Work out the finished part from the listing and answer in its coordinate system (mm). A direction names the side the tool comes from. Give positions to 0.01 mm unless a question says otherwise; leave off trailing zeros. Loops run counter-clockwise (first coordinate to the right, second up) from the corner with the lowest first, then second, coordinate; pieces in that order, holes last. Notation, with made-up numbers: (82, -12.5) - (112, -12.5) arc R22 cw to (112, 11.5) - close; hole circle Ø8 at (21, 26). An arc over 180 degrees is marked (long way). One line per question, with ' | ' between items. Start each with the question number.
1. For a pull along X with two mould halves and no side action, classify faces 1 (the face through (-5, -1.5, 2)), 2 (the face through (7.5, 0, 3)), 3 (the face through (0, -7.5, 3)) as released by +X, released by -X, zero draft, split by the parting line, or undercut.
2. Section B-B (z = 2.15) is taken. Determine the outline of the cut face in (x, y), plus the area to 3 significant figures.
3. Which of the six approach directions +Z, -Z, +X, -X, +Y, -Y give full straight-line access (tool end or side, diameter ignored) to faces 4 (the face through (0, 0, 6)), 5 (the face through (5.55, -3, 2))?
4. Find the intervals of material crossed by line 1 (Y direction, x = -5.5, z = 3.55); line 2 (Y direction, x = 0, z = 4.4), in increasing order.
5. Section D-D (y = 0) is taken. Determine the outline of the cut face in (x, z).
6. Section A-A (x = -5.25) is taken. Determine the outline of the cut face in (y, z).
from build123d import *

# Parameters (mm, degrees)
SKETCH1_W           = 15
SKETCH1_H           = 15
BOSS_EXTRUDE1_DEPTH = 5
SKETCH2_W           = 15
SKETCH2_H           = 15
BOSS_EXTRUDE2_DEPTH = 1


with BuildPart() as part:
    # Sketch1 → Boss-Extrude1 (new body)
    with BuildSketch(Plane.XY):
        Rectangle(SKETCH1_W, SKETCH1_H)
        Polygon((-5.55, 5.55), (-1.5, 5.55), (-1.5, 3.55), (1.5, 3.55), (1.5, 5.55), (5.55, 5.55), (5.55, 1.5), (3.55, 1.5), (3.55, -1.5), (5.55, -1.5), (5.55, -5.55), (1.5, -5.55), (1.5, -3.55), (-1.5, -3.55), (-1.5, -5.55), (-5.55, -5.55), (-5.55, -1.5), (-3.55, -1.5), (-3.55, 1.5), (-5.55, 1.5), align=None, mode=Mode.SUBTRACT)
    extrude(amount=BOSS_EXTRUDE1_DEPTH)

    # Sketch2 → Boss-Extrude2 (add)
    with BuildSketch(Plane.XY.offset(5)):
        Rectangle(SKETCH2_W, SKETCH2_H)
    extrude(amount=BOSS_EXTRUDE2_DEPTH)


solid = part.part
Conclusion:
1) face 1: undercut | face 2: released by +X | face 3: zero draft
2) outline: (-7.5, -7.5) - (7.5, -7.5) - (7.5, 7.5) - (-7.5, 7.5) - close; hole (-5.55, -5.55) - (-1.5, -5.55) - (-1.5, -3.55) - (1.5, -3.55) - (1.5, -5.55) - (5.55, -5.55) - (5.55, -1.5) - (3.55, -1.5) - (3.55, 1.5) - (5.55, 1.5) - (5.55, 5.55) - (1.5, 5.55) - (1.5, 3.55) - (-1.5, 3.55) - (-1.5, 5.55) - (-5.55, 5.55) - (-5.55, 1.5) - (-3.55, 1.5) - (-3.55, -1.5) - (-5.55, -1.5) - close | area: 126 mm²
3) face 4: +Z, +X, -X, +Y, -Y | face 5: -Z
4) line 1: -7.5 to -5.55, -1.5 to 1.5, 5.55 to 7.5 | line 2: -7.5 to -3.55, 3.55 to 7.5
5) outline: (-7.5, 0) - (-3.55, 0) - (-3.55, 5) - (3.55, 5) - (3.55, 0) - (7.5, 0) - (7.5, 6) - (-7.5, 6) - close
6) outline: (-7.5, 0) - (-5.55, 0) - (-5.55, 5) - (-1.5, 5) - (-1.5, 0) - (1.5, 0) - (1.5, 5) - (5.55, 5) - (5.55, 0) - (7.5, 0) - (7.5, 6) - (-7.5, 6) - close
